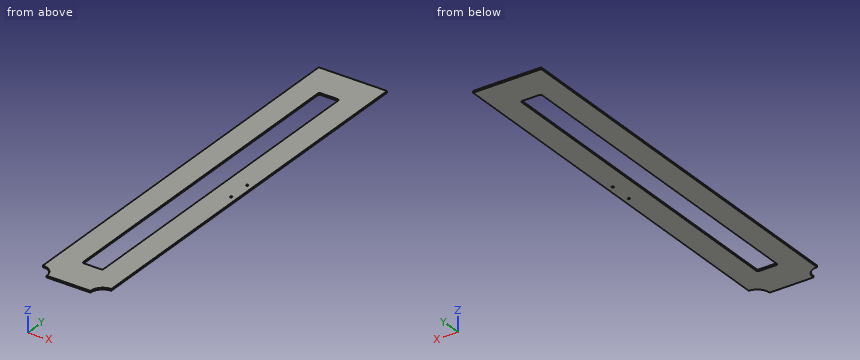
```python
from build123d import *

# Parameters (mm, degrees)
SKETCH1_W           = 200
SKETCH1_H           = 1200
BOSS_EXTRUDE1_DEPTH = 5
CUT_EXTRUDE1_DEPTH  = 609.296802556
SKETCH5_W           = 60
SKETCH5_H           = 1000
CUT_EXTRUDE3_DEPTH  = 609.296802556
FILLET2_R           = 5
SKETCH6_R           = 3
CUT_EXTRUDE4_DEPTH  = 609.296802556


with BuildPart() as part:
    # Sketch1 → Boss-Extrude1 (new body)
    with BuildSketch(Plane.XY):
        Rectangle(SKETCH1_W, SKETCH1_H)
    extrude(amount=BOSS_EXTRUDE1_DEPTH)

    # Sketch3 → Cut-Extrude1 (cut, through all)
    with BuildSketch(Plane.XY.offset(5)):
        with BuildLine():
            Line((-100, -600), (-100, -564.197190266))
            ThreePointArc((-100, -564.197190266), (-74.683590452, -574.683590452), (-64.197190266, -600))
            Line((-64.197190266, -600), (-100, -600))
        make_face()
        with BuildLine():
            Line((64.197190266, -600), (100, -600))
            Line((100, -600), (100, -564.197190266))
            ThreePointArc((100, -564.197190266), (74.683590452, -574.683590452), (64.197190266, -600))
        make_face()
    extrude(amount=-CUT_EXTRUDE1_DEPTH, mode=Mode.SUBTRACT)

    # Sketch5 → Cut-Extrude3 (cut, through all)
    with BuildSketch(Plane.XY.offset(5)):
        Rectangle(SKETCH5_W, SKETCH5_H)
    extrude(amount=-CUT_EXTRUDE3_DEPTH, mode=Mode.SUBTRACT)

    # Fillet2
    fillet2_edges = [part.edges().sort_by_distance(p)[0] for p in [
        (30, 500, 2.5),
        (30, -500, 2.5),
        (-30, -500, 2.5),
        (-30, 500, 2.5),
    ]]
    fillet(fillet2_edges, radius=FILLET2_R)

    # Sketch6 → Cut-Extrude4 (cut, through all)
    with BuildSketch(Plane.XY.offset(5)):
        with Locations((83.193225438, -34)):
            Circle(SKETCH6_R)
        with Locations((83.193225438, 34)):
            Circle(SKETCH6_R)
    extrude(amount=-CUT_EXTRUDE4_DEPTH, mode=Mode.SUBTRACT)


solid = part.part
```
CAD build for the part. Positions are in the model's coordinates, mm. Round coordinates to 2 decimals unless told otherwise and drop trailing zeros. Order: outer loops, then holes, each group sorted by start corner. A loop starts at its lowest first (then second) coordinate and runs counter-clockwise, first axis right, second up.
Q1. Slice it at C-C (z = 3.7). Write the cut outline in (x, y), and give its area (3 significant figures).
Q2. Slice it at A-A (x = 7). Write the cut outline in (y, z), and give its area (3 significant figures).
Q3. Drop a flat-ended pin along its axis: pin 1 (3.5 mm diameter, centred on x = 83.19, y = -34, fed in from -Z). Give the stop position or say it passes through.
Q4. Wall check: L1, parallel to Y at x = -10, z = 3.45; L2, parallel to X at y = -229.5, z = 2.1; L3, parallel to Y at x = -69.5, z = 2. Give the ranges that are in metal, low to high.
Q5. Slice it at B-B (y = 348.5). Write the cut outline in (x, z).
Results below:
1. outline: (-100, -564.2) arc R35.8 cw to (-64.2, -600) - (64.2, -600) arc R35.8 cw to (100, -564.2) - (100, 600) - (-100, 600) - close; hole (-30, -495) arc R5 ccw to (-25, -500) - (25, -500) arc R5 ccw to (30, -495) - (30, 495) arc R5 ccw to (25, 500) - (-25, 500) arc R5 ccw to (-30, 495) - close; hole circle Ø6 at (83.19, -34); hole circle Ø6 at (83.19, 34)
1. area: 178,000 mm2
2. outline: (-600, 0) - (-500, 0) - (-500, 5) - (-600, 5) - close; (500, 0) - (600, 0) - (600, 5) - (500, 5) - close
2. area: 1,000 mm2
3. pin 1: passes through
4. L1: y = -600 to -500, 500 to 600
4. L2: x = -100 to -30, 30 to 100
4. L3: y = -581.25 to 600
5. outline: (-100, 0) - (-30, 0) - (-30, 5) - (-100, 5) - close; (30, 0) - (100, 0) - (100, 5) - (30, 5) - close
